from build123d import *

# Parameters (mm, degrees)
SKETCH1_W           = 965.2
SKETCH1_H           = 812.8
SKETCH1_W_2         = 812.8
SKETCH1_H_2         = 660.4
BOSS_EXTRUDE1_DEPTH = 127
FILLET1_R           = 17.78


with BuildPart() as part:
    # Sketch1 → Boss-Extrude1 (new body)
    with BuildSketch(Plane(origin=(0, 0, 0), x_dir=(1, 0, 0), z_dir=(0, 1, 0))):
        Rectangle(SKETCH1_W, SKETCH1_H)
        Rectangle(SKETCH1_W_2, SKETCH1_H_2, mode=Mode.SUBTRACT)
    extrude(amount=BOSS_EXTRUDE1_DEPTH)

    # Fillet1
    fillet1_edges = [part.edges().sort_by_distance(p)[0] for p in [
        (482.6, 127, 0),
        (406.4, 127, 0),
        (0, 127, -406.4),
        (0, 127, -330.2),
        (-406.4, 127, 0),
        (0, 127, 330.2),
        (-482.6, 127, 0),
        (0, 0, -406.4),
        (482.6, 0, 0),
        (0, 0, 406.4),
        (-482.6, 0, 0),
        (0, 127, 406.4),
    ]]
    fillet(fillet1_edges, radius=FILLET1_R)


solid = part.part
For this review, take the finished solid that the model builds, in its own axes (mm). A direction names the side the tool comes from. Round coordinates to 2 decimals unless told otherwise and drop trailing zeros. Order: outer loops, then holes, each group sorted by start corner. A loop starts at its lowest first (then second) coordinate and runs counter-clockwise, first axis right, second up. Notation, with made-up numbers: (78, 47.25) -> (131, 47.25) arc R30 ccw to (131, 82.25) -> close; hole circle Ø8 at (11.5, 49.25). An arc over 180 degrees is marked (long way). Write item = value, one per line. Start each with the question number.
1) Take a section at B-B on x = 309.5. State the section outline as (y, z) points.
2) Tool access review of faces 4 (the face through (406.4, 54, 5)), 5 (the face through (-7, 0, 340)): name each direction out of +Z, -Z, +X, -X, +Y, -Y from which nothing blocks a thin tool from reaching the whole face with its end or side.
3) Take a section at A-A on z = 227.5. State the section outline as (x, y) points, plus the area to 3 significant figures.
4) Take a section at C-C on y = 96.5. State the section outline as (x, z) points.
5) The part is to be moulded in two halves that separate along Z. For faces 1 (the face through (-6, 54, -330.2)), 2 (the face through (-482.6, 63, 6)), 3 (the face through (-7, 63, -406.4)), say which applies: +Z half, -Z half, draft (parallel to the pull), parting line (faces both ways), or undercut.
6) To check wall thickness, follow line 1 (X direction, y = 72, z = -263); line 2 (Z direction, x = 224.5, y = 84); line 3 (X direction, y = 116, z = -54.5). State the ranges of each line that lie inside material, in increasing order. Write a range as from..to.
Verdict:
q1.outline = (0, -388.62) arc R17.78 ccw to (17.78, -406.4) -> (109.22, -406.4) arc R17.78 ccw to (127, -388.62) -> (127, -347.98) arc R17.78 ccw to (109.22, -330.2) -> (0, -330.2) -> close; (0, 330.2) -> (109.22, 330.2) arc R17.78 ccw to (127, 347.98) -> (127, 388.62) arc R17.78 ccw to (109.22, 406.4) -> (17.78, 406.4) arc R17.78 ccw to (0, 388.62) -> close
q2.face_4 = +Y, -Y
q2.face_5 = +Z, -Z, +X, -X, -Y
q3.outline = (-482.6, 17.78) arc R17.78 ccw to (-464.82, 0) -> (-406.4, 0) -> (-406.4, 109.22) arc R17.78 ccw to (-424.18, 127) -> (-464.82, 127) arc R17.78 ccw to (-482.6, 109.22) -> close; (406.4, 0) -> (464.82, 0) arc R17.78 ccw to (482.6, 17.78) -> (482.6, 109.22) arc R17.78 ccw to (464.82, 127) -> (424.18, 127) arc R17.78 ccw to (406.4, 109.22) -> close
q3.area = 18,900 mm2
q4.outline = (-482.6, -406.4) -> (482.6, -406.4) -> (482.6, 406.4) -> (-482.6, 406.4) -> close; hole (-406.4, -330.2) -> (406.4, -330.2) -> (406.4, 330.2) -> (-406.4, 330.2) -> close
q5.face_1 = undercut
q5.face_2 = draft
q5.face_3 = -Z half
q6.line_1 = -482.6..-406.4, 406.4..482.6
q6.line_2 = -406.4..-330.2, 330.2..406.4
q6.line_3 = -481.26..-407.74, 407.74..481.26
